Part model, mm, in its own coordinate system. A direction names the side the tool comes from. Give positions to 0.01 mm unless a question says otherwise; leave off trailing zeros. Order: outer loops, then holes, each group sorted by start corner. A loop starts at its lowest first (then second) coordinate and runs counter-clockwise, first axis right, second up.
from build123d import *

# Parameters (mm, degrees)
CYLINDER271_R               = 8
CYLINDER271_DEPTH           = 6
CYLINDER271_PLACEMENT_ANGLE = 240
CYLINDER272_R               = 3
CYLINDER272_DEPTH           = 3
CYLINDER232_R               = 3
CYLINDER232_DEPTH           = 3
COMPOUND244_PLACEMENT_ANGLE = 240
COMPOUND214_PLACEMENT_ANGLE = 120
CYLINDER233_R               = 1.5
CYLINDER233_DEPTH           = 60
CYLINDER234_R               = 1.5
CYLINDER234_DEPTH           = 60
COMPOUND240_PLACEMENT_ANGLE = 240
COMPOUND215_PLACEMENT_ANGLE = 120
CYLINDER268_R               = 15
CYLINDER268_DEPTH           = 20
CYLINDER269_R               = 8
CYLINDER269_DEPTH           = 6
CYLINDER269_PLACEMENT_ANGLE = 120
CYLINDER231_R               = 8
CYLINDER231_DEPTH           = 6
CYLINDER231_PLACEMENT_ANGLE = 240
CYLINDER270_R               = 8
CYLINDER270_DEPTH           = 6
CYLINDER267_R               = 40
CYLINDER267_DEPTH           = 8


with BuildPart() as obj1:
    # Cylinder271 → Cylinder271 (new body)
    with BuildSketch(Plane.XY):
        Circle(CYLINDER271_R)
    extrude(amount=CYLINDER271_DEPTH)


with BuildPart() as obj1_1:
    # Cylinder271 placement: moved
    add(obj1.part.moved(Location((0, 0, 2))).rotate(Axis((0, 0, 2), (0, 0, 1)), CYLINDER271_PLACEMENT_ANGLE))


with BuildPart() as obj2:
    # Cylinder272 → Cylinder272 (new body)
    with BuildSketch(Plane(origin=(29, -5, -6), x_dir=(1, 0, 0), z_dir=(0, 0, 1))):
        Circle(CYLINDER272_R)
    extrude(amount=CYLINDER272_DEPTH)


with BuildPart() as obj3:
    # Cylinder232 → Cylinder232 (new body)
    with BuildSketch(Plane(origin=(29, 5, -6), x_dir=(1, 0, 0), z_dir=(0, 0, 1))):
        Circle(CYLINDER232_R)
    extrude(amount=CYLINDER232_DEPTH)


with BuildPart() as compound244:
    # Compound244 base: copy of obj3
    add(obj3.part)

    # Compound244: union obj2
    add(obj2.part)


with BuildPart() as compound244_1:
    # Compound244 placement: moved
    add(compound244.part.moved(Location((0, 0, 6))).rotate(Axis((0, 0, 6), (0, 0, 1)), COMPOUND244_PLACEMENT_ANGLE))


with BuildPart() as compound246:
    # Compound246 base: copy of obj3
    add(obj3.part)

    # Compound246: union obj2
    add(obj2.part)


with BuildPart() as compound246_1:
    # Compound246 placement: moved
    add(compound246.part.moved(Location((0, 0, 6))))


with BuildPart() as compound242:
    # Compound214 base: copy of obj3
    add(obj3.part)

    # Compound214: union obj2
    add(obj2.part)


with BuildPart() as compound242_1:
    # Compound214 placement: moved
    add(compound242.part.moved(Location((0, 0, 6))).rotate(Axis((0, 0, 6), (0, 0, 1)), COMPOUND214_PLACEMENT_ANGLE))

    # Compound242: union Compound244, Compound246
    add(compound244_1.part)
    add(compound246_1.part)


with BuildPart() as obj4:
    # Cylinder233 → Cylinder233 (new body)
    with BuildSketch(Plane(origin=(29, -5, -6), x_dir=(1, 0, 0), z_dir=(0, 0, 1))):
        Circle(CYLINDER233_R)
    extrude(amount=CYLINDER233_DEPTH)


with BuildPart() as obj5:
    # Cylinder234 → Cylinder234 (new body)
    with BuildSketch(Plane(origin=(29, 5, -6), x_dir=(1, 0, 0), z_dir=(0, 0, 1))):
        Circle(CYLINDER234_R)
    extrude(amount=CYLINDER234_DEPTH)


with BuildPart() as compound240:
    # Compound240 base: copy of obj5
    add(obj5.part)

    # Compound240: union obj4
    add(obj4.part)


with BuildPart() as compound240_1:
    # Compound240 placement: moved
    add(compound240.part.rotate(Axis((0, 0, 0), (0, 0, 1)), COMPOUND240_PLACEMENT_ANGLE))


with BuildPart() as compound243:
    # Compound243 base: copy of obj5
    add(obj5.part)

    # Compound243: union obj4
    add(obj4.part)


with BuildPart() as compound238:
    # Compound215 base: copy of obj5
    add(obj5.part)

    # Compound215: union obj4
    add(obj4.part)


with BuildPart() as compound238_1:
    # Compound215 placement: moved
    add(compound238.part.rotate(Axis((0, 0, 0), (0, 0, 1)), COMPOUND215_PLACEMENT_ANGLE))

    # Compound238: union Compound240, Compound243
    add(compound240_1.part)
    add(compound243.part)


with BuildPart() as obj6:
    # Cylinder268 → Cylinder268 (new body)
    with BuildSketch(Plane.XY.offset(-100)):
        Circle(CYLINDER268_R)
    extrude(amount=CYLINDER268_DEPTH)


with BuildPart() as obj7:
    # Cylinder269 → Cylinder269 (new body)
    with BuildSketch(Plane.XY):
        Circle(CYLINDER269_R)
    extrude(amount=CYLINDER269_DEPTH)


with BuildPart() as obj7_1:
    # Cylinder269 placement: moved
    add(obj7.part.moved(Location((12.5, -21.65, 2))).rotate(Axis((12.5, -21.65, 2), (0, 0, 1)), CYLINDER269_PLACEMENT_ANGLE))


with BuildPart() as obj8:
    # Cylinder231 → Cylinder231 (new body)
    with BuildSketch(Plane.XY):
        Circle(CYLINDER231_R)
    extrude(amount=CYLINDER231_DEPTH)


with BuildPart() as obj8_1:
    # Cylinder231 placement: moved
    add(obj8.part.moved(Location((12.5, 21.65, 2))).rotate(Axis((12.5, 21.65, 2), (0, 0, 1)), CYLINDER231_PLACEMENT_ANGLE))


with BuildPart() as compound239:
    # Cylinder270 → Cylinder270 (new body)
    with BuildSketch(Plane(origin=(-25, 0, 2), x_dir=(1, 0, 0), z_dir=(0, 0, 1))):
        Circle(CYLINDER270_R)
    extrude(amount=CYLINDER270_DEPTH)

    # Compound239: union obj7, obj8
    add(obj7_1.part)
    add(obj8_1.part)


with BuildPart() as cut116:
    # Cylinder267 → Cylinder267 (new body)
    with BuildSketch(Plane.XY):
        Circle(CYLINDER267_R)
    extrude(amount=CYLINDER267_DEPTH)

    # Cut113: cut Compound239
    add(compound239.part, mode=Mode.SUBTRACT)

    # Cut112: cut obj6
    add(obj6.part, mode=Mode.SUBTRACT)

    # Cut114: cut Compound238
    add(compound238_1.part, mode=Mode.SUBTRACT)

    # Cut115: cut Compound242
    add(compound242_1.part, mode=Mode.SUBTRACT)

    # Cut116: cut obj1
    add(obj1_1.part, mode=Mode.SUBTRACT)


solid = cut116.part
Item 1: Band-saw the part on D-D on y = 0. List the corners of the cut face in (x, z), plus the area to 3 significant figures.
Item 2: Pull direction X, two halves, no side cores. Call faces 1 (the face through (-0.6, -8.3, 8)), 2 (the face through (-20, 21, 3)): released by +X, released by -X, zero draft, split by the parting line, or undercut.
Item 3: Band-saw the part on B-B on z = 4. Give the number of separate pieces and of enclosed holes in the cut face, plus the area to 3 significant figures.
Item 4: Which spindle directions (+Z, -Z, +X, -X, +Y, -Y) get a long thin tool onto all of the face, cutting with end or side? Do faces 3 (the face through (-17, -23, 3)), 4 (the face through (7.63, 2.4, 4.96)), 5 (the face through (-11.275, -26.601, 5.465)). Say none if no direction does.
Item 5: Band-saw the part on A-A on y = -28. List the corners of the cut face in (x, z), plus the area to 3 significant figures.
Item 6: Drop flat-ended pins along their axis: P1, Ø5, axis at x = -18.83, y = 22.61, coming from the -Z side; P2, Ø3, axis at x = 5.5, z = 1, coming from the +Y side; P3, Ø1.8, axis at x = -10.17, y = 27.61, coming from the -Z side; P4, Ø1, axis at x = 23, z = 3.5, coming from the +Y side. Give the stop position or say it passes through.
Item 7: Drill centre lines: probe 1 along Y at (x, z) = (28, 7.25); probe 2 along Y at (x, z) = (14, 7); probe 3 along Y at (x, z) = (0, 3.5). Where is each one in solid material? Low to high.
Item 8: Band-saw the part on C-C on x = 12.5. List the corners of the cut face in (y, z).
Working result:
1. outline: (-40, 0) - (40, 0) - (40, 8) - (8, 8) - (8, 2) - (-8, 2) - (-8, 8) - (-17, 8) - (-17, 2) - (-33, 2) - (-33, 8) - (-40, 8) - close
1. area: 448 mm2
2. face 1: zero draft
2. face 2: undercut
3. separate pieces: 1
3. enclosed holes: 10
3. area: 4,180 mm2
4. face 3: -Z
4. face 4: +Z
4. face 5: +Z, -Z
5. outline: (-28.57, 0) - (-13.15, 0) - (-13.15, 3) - (-11.62, 3) - (-11.62, 8) - (-28.57, 8) - close; (-8.72, 3) - (-7.19, 3) - (-7.19, 0) - (28.57, 0) - (28.57, 8) - (17.37, 8) - (17.37, 2) - (7.63, 2) - (7.63, 8) - (-8.72, 8) - close
5. area: 366 mm2
6. P1: stops at z = 3
6. P2: stops at y = 39.8
6. P3: passes through
6. P4: stops at y = 33.07
7. probe 1: y = -28.57 to -6.12, -3.88 to 3.88, 6.12 to 28.57
7. probe 2: y = -37.47 to -29.51, -13.79 to 13.79, 29.51 to 37.47
7. probe 3: y = -40 to -8, 8 to 40
8. outline: (-38, 0) - (38, 0) - (38, 8) - (29.65, 8) - (29.65, 2) - (13.65, 2) - (13.65, 8) - (-13.65, 8) - (-13.65, 2) - (-29.65, 2) - (-29.65, 8) - (-38, 8) - close
